Geometry: see drawing. Coordinates: mm, zero at the bounding-box minimum. Give positions to 0.01 mm unless a question says otherwise; leave off trailing zeros. Order: outer loops, then holes, each group sorted by start corner. A loop starts at its lowest first (then second) coordinate and runs counter-clockwise, first axis right, second up. Notation, with made-up numbers: M 2,46 L 33,46 A29 cw 33,77 Z; hole C -16,63.5 d2. An arc over 180 degrees is marked long. Use a Markdown table: item, result.
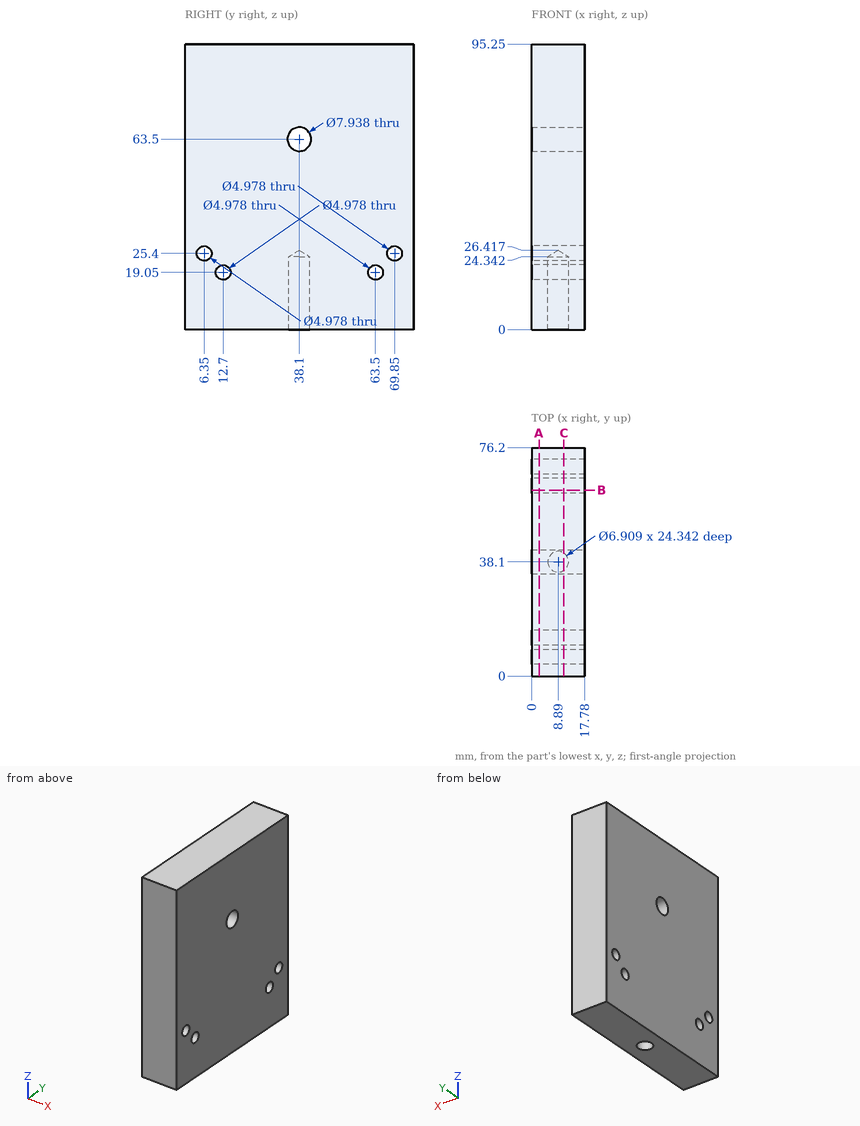
1) Cut plane A-A on x = 2.5. Return loops of the section in (y, z).
Response values:
| item | result |
|---|---|
| outline | M 0,0 L 76.2,0 L 76.2,95.25 L 0,95.25 Z; hole C 6.35,25.4 d4.98; hole C 12.7,19.05 d4.98; hole C 38.1,63.5 d7.94; hole C 63.5,19.05 d4.98; hole C 69.85,25.4 d4.98 |
2) Cut plane B-B on y = 62. Return loops of the section in (x, z), and give its area (3 significant figures).
Response values:
| item | result |
|---|---|
| outline | M 0,0 L 17.78,0 L 17.78,17.06 L 0,17.06 Z; M 0,21.04 L 17.78,21.04 L 17.78,95.25 L 0,95.25 Z |
| area | 1,620 mm² |
3) Cut plane C-C on x = 10.75. State how many separate pieces and enclosed holes the cut face has, and give its area (3 significant figures).
Response values:
| item | result |
|---|---|
| separate pieces | 1 |
| enclosed holes | 5 |
| area | 6,990 mm² |
4) Material intervals for line 1 (Z direction, x = 10.75, y = 6.35); line 2 (Z direction, x = 13.25, y = 12.7); line 3 (Y direction, x = 15.5, z = 66.5) (1 decimal), sorted ascending. Write a range as from..to.
Response values:
| item | result |
|---|---|
| line 1 | z = 0..22.91, 27.89..95.25 |
| line 2 | z = 0..16.56, 21.54..95.25 |
| line 3 | y = 0..35.5, 40.7..76.2 |
